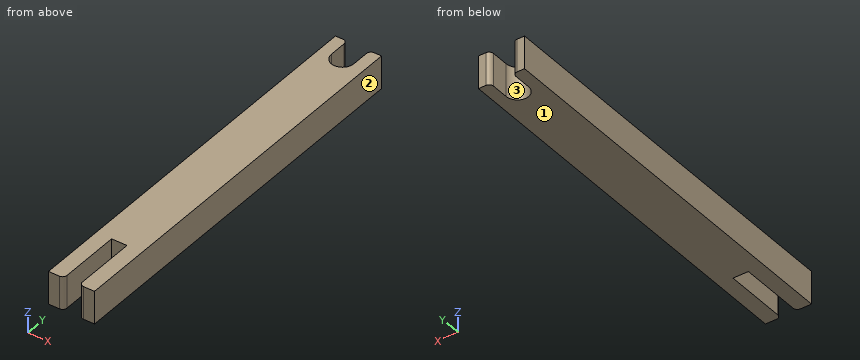
from build123d import *

# Parameters (mm, degrees)
F1_DEPTH = 7.5
F2_R     = 2


with BuildPart() as f1:
    # F0 (on Top) → F1 (new body, symmetric)
    with BuildSketch(Plane.XY):
        with BuildLine():
            Line((3.5, -90.05), (10.5, -90.05))
            Line((10.5, -90.05), (10.5, 90.05))
            Line((10.5, 90.05), (5.1, 90.05))
            Line((5.1, 90.05), (5.1, 80.05))
            ThreePointArc((5.1, 80.05), (0, 74.95), (-5.1, 80.05))
            Line((-5.1, 80.05), (-5.1, 90.05))
            Line((-5.1, 90.05), (-10.5, 90.05))
            Line((-10.5, 90.05), (-10.5, -90.05))
            Line((-10.5, -90.05), (-3.5, -90.05))
            Line((-3.5, -90.05), (-3.5, -60.05))
            Line((-3.5, -60.05), (3.5, -60.05))
            Line((3.5, -60.05), (3.5, -90.05))
        make_face()
    extrude(amount=F1_DEPTH, both=True)

    # F2
    f2_edges = [f1.edges().sort_by_distance(p)[0] for p in [
        (5.1, 90.05, 0),
        (-5.1, 90.05, 0),
        (-3.5, -90.05, 0),
        (3.5, -90.05, 0),
    ]]
    fillet(f2_edges, radius=F2_R)


solid = f1.part
Here's how the part is built. I have some questions about the finished solid (model axes, mm). Face numbers are marked on the shaded views. Round coordinates to 2 decimals unless told otherwise and drop trailing zeros. Write each loop counter-clockwise with the first axis right and the second up, starting at its lowest first coordinate (ties: lowest second). Pieces come first, ordered by that corner, then holes.
1. If we mould it in two halves opening along X, with no side actions, what happens to the marked faces 1, 2 and 3? For each: released by +X, released by -X, zero draft, split by the parting line, or undercut.
2. I need wall thicknesses on L1, parallel to X at y = -79.5, z = 5.75; L2, parallel to Y at x = -0.5, z = -2.5; L3, parallel to X at y = 76, z = 0.5. Which ranges of each line are inside material? Lowest first, please.
3. Will this pin go through, and if not, where does the flat tip stop? pin 1 Ø2 at (x, z) = (-0.5, 0) entering from -Y.
4. Suppose I cut it at B-B (x = 0). List the corners of the cut face in (y, z) for me.
5. Suppose I cut it at A-A (z = -5). List the corners of the cut face in (x, y) for me, and give its area (3 significant figures).
Answer sheet:
1. face 1: zero draft
1. face 2: released by +X
1. face 3: undercut
2. L1: x = -10.5 to -3.5, 3.5 to 10.5
2. L2: y = -60.05 to 74.97
2. L3: x = -10.5 to -3.1, 3.1 to 10.5
3. pin 1: stops at y = -60.05
4. outline: (-60.05, -7.5) - (74.95, -7.5) - (74.95, 7.5) - (-60.05, 7.5) - close
5. outline: (-10.5, -90.05) - (-5.5, -90.05) arc R2 ccw to (-3.5, -88.05) - (-3.5, -60.05) - (3.5, -60.05) - (3.5, -88.05) arc R2 ccw to (5.5, -90.05) - (10.5, -90.05) - (10.5, 90.05) - (7.1, 90.05) arc R2 ccw to (5.1, 88.05) - (5.1, 80.05) arc R5.1 cw to (-5.1, 80.05) - (-5.1, 88.05) arc R2 ccw to (-7.1, 90.05) - (-10.5, 90.05) - close
5. area: 3,430 mm2
